Autodesk Inventor part; units mm, degrees
ref_plane "YZ Plane" through (0, 0, 0) normal (1, 0, 0) x (0, 1, 0)
ref_plane "XZ Plane" through (0, 0, 0) normal (0, 1, 0) x (-1, 0, 0)
ref_plane "XY Plane" through (0, 0, 0) normal (0, 0, 1) x (1, 0, 0)
sketch "Sketch1" plane through (0, 0, 0) normal (0, 1, 0) x (-1, 0, 0)
  line L0 (-26, 23.75) -> (26, 23.75)
  line L1 (26, 23.75) -> (26, -23.75)
  line L2 (26, -23.75) -> (-26, -23.75)
  line L3 (-26, -23.75) -> (-26, 23.75)
  line L4 (-26, 23.75) -> (26, -23.75) construction
  line L5 (26, 23.75) -> (-26, -23.75) construction
  point P0 (0, 0)
  dimension "d0" = 52
  dimension "d1" = 47.5
extrude "Extrusion1" add sketch "Sketch1" along normal blind 3
fillet "Fillet1" radius 5 2 edges at (26, 1.5, 23.75) (-26, 1.5, 23.75)
sketch "Sketch2" plane through (0, 3, 0) normal (0, 1, 0) x (1, 0, 0)
  arc A0 (-26, -18.75) -> (-21, -23.75) centre (-21, -18.75) ccw
  line L0 (-21, -23.75) -> (21, -23.75)
  arc A1 (21, -23.75) -> (26, -18.75) centre (21, -18.75) ccw
  line L1 (26, -18.75) -> (26, 23.75)
  line L2 (26, 23.75) -> (-26, 23.75)
  line L3 (-26, 23.75) -> (-26, -18.75)
  line L4 (29, 26.75) -> (29, -18.75)
  arc A2 (21, -26.75) -> (29, -18.75) centre (21, -18.75) ccw
  line L5 (21, -26.75) -> (-21, -26.75)
  arc A3 (-29, -18.75) -> (-21, -26.75) centre (-21, -18.75) ccw
  line L6 (-29, -18.75) -> (-29, 26.75)
  line L7 (-29, 26.75) -> (29, 26.75)
  point P0 (0, 0)
  dimension "d5" = 3
extrude "Extrusion2" add sketch "Sketch2" against normal blind 5
sketch "Sketch3" plane through (0, 3, 0) normal (0, 1, 0) x (1, 0, 0)
  line L0 (26, -18.75) -> (26, 23.75)
  line L1 (29, 26.75) -> (26, 26.75)
  line L2 (26, 26.75) -> (26, 23.75)
  line L3 (26, 23.75) -> (29, 23.75)
  line L4 (29, 23.75) -> (29, 26.75)
  line L5 (26, 23.75) -> (21, 23.75)
  line L6 (21, 23.75) -> (21, 18.75)
  line L7 (21, 18.75) -> (26, 18.75)
  line L8 (26, 18.75) -> (26, 23.75)
  line L9 (-29, 26.75) -> (-26, 26.75)
  line L10 (-26, 26.75) -> (-26, 23.75)
  line L11 (-26, 23.75) -> (-29, 23.75)
  line L12 (-29, 23.75) -> (-29, 26.75)
  line L13 (-26, 23.75) -> (-21, 23.75)
  line L14 (-21, 23.75) -> (-21, 18.75)
  line L15 (-21, 18.75) -> (-26, 18.75)
  line L16 (-26, 18.75) -> (-26, 23.75)
  arc A0 (-29, -18.75) -> (-21, -26.75) centre (-21, -18.75) ccw
  line L17 (21, 18.75) -> (-21, 18.75)
  line L18 (-21, 18.75) -> (-21, -18.75)
  line L19 (-21, -18.75) -> (21, -18.75)
  line L20 (21, -18.75) -> (21, 18.75)
  line L21 (-21, -18.75) -> (-26, -18.75)
  line L22 (-26, -18.75) -> (-26, -23.75)
  line L23 (-26, -23.75) -> (-21, -23.75)
  line L24 (-21, -23.75) -> (-21, -18.75)
  line L25 (-21, -18.75) -> (-24.5355, -22.2855)
  line L26 (-21, -18.75) -> (-16, -18.75) construction
  line L27 (21, -18.75) -> (24.5355, -22.2855)
  line L28 (24.5355, -22.2855) -> (-24.5355, -22.2855)
  line L29 (26, 18.75) -> (21, 23.75)
  line L30 (-21, 23.75) -> (-26, 18.75)
  line L31 (22.7678, -20.5178) -> (-22.7678, -20.5178)
  line L32 (23.5, 21.25) -> (-23.5, 21.25)
  point P0 (0, 0)
  dimension "d8" = 3
  dimension "d9" = 3
  dimension "d10" = 5
  dimension "d11" = 5
  dimension "d12" = 3
  dimension "d13" = 3
  dimension "d14" = 5
  dimension "d15" = 5
  dimension "d16" = 37.5
  dimension "d17" = 5
  dimension "d18" = 5
  dimension "d19" = 5
  dimension "d20" = 135
  dimension "d21" = 5
hole "Hole1" at (-23.5, 3, -21.25) at (23.5, 3, -21.25) at (22.7678, 3, 20.5178) at (-22.7678, 3, 20.5178) direction (0, -1, 0) diameter 2.2 end through all countersink diameter 4 countersink angle 90
fillet "Fillet2" radius 3 5 edges at (26.6569, 3, 24.4069) (0, 3, 26.75) (-26.6569, 3, 24.4069) (-29, 3, -4) (29, 3, -4)
thicken "Thicken1" operation add thickness 3 both sides no extend neighbours yes toward (0, 0, 1) faces at (8.6667, -0.3333, -26.75)
properties part number "Closing_Stepper_2"
Input: part model. Units: mm. Frame: model coordinates. A direction names the side the tool comes from. Round coordinates to 2 decimals unless told otherwise and drop trailing zeros. Loops run counter-clockwise (first coordinate to the right, second up) from the corner with the lowest first, then second, coordinate; pieces in that order, holes last. Notation, with made-up numbers: M -24,2 L 28,2 A16 cw 28,10 Z; hole C 51.5,66 d2. An arc over 180 degrees is marked long. Answer as CSV lines item,"result". Start each with the question number.
(1) First-contact query: pin 1 (2.5 mm diameter, centred on x = 22.77, z = 20.52, fed in from +Y); pin 2 (0.6 mm diameter, centred on x = 0.5, y = -1.5, fed in from -Z); pin 3 (1 mm diameter, centred on x = -20.5, z = 10.5, fed in from -Y). Flat tips, straight axial feed; report the tip coordinate or a pass-through.
(2) Section C-C, the plane y = 0.9. Output: boundary loops of the cut face in (x, z), plus the area to 3 significant figures.
(3) Section B-B, the plane x = 15. Output: boundary loops of the cut face in (y, z).
(4) Section D-D, the plane z = -14. Output: boundary loops of the cut face in (x, y).
(5) Draft query along X for faces 3 (the cylindrical face through (-28.1, 2.14, -2.2)), 4 (the flat face through (0, -1, 23.75)), 5 (the flat face through (29, -1, -3)). Return one class per face: released by +X, released by -X, zero draft, split by the parting line, or undercut.
(6) Section A-A, the plane z = -21.25. Output: boundary loops of the cut face in (x, y), plus the area to 3 significant figures.
(7) Line query: line 1 (X direction, y = 0.45, z = -21.25); line 2 (X direction, y = -1.55, z = -4); line 3 (Y direction, x = -1, z = -7). Output: solid intervals per line, ascending. Write a range as [from, to].
(8) Reachability of faces 1 (the flat face through (0, 2, -23.75)), 2 (the cylindrical face through (-24.57, -0.99, 22.25)) from +Z, -Z, +X, -X, +Y, -Y: full face, straight path, thin tool, end or side. Return the list, or none.
Values found:
1,pin 1,"stops at y = 2.25"
1,pin 2,"stops at z = 23.75"
1,pin 3,"stops at y = 0"
2,outline,"M -28.86,-23.75 L 28.86,-23.75 L 28.86,18.75 A7.86 ccw 21,26.61 L -21,26.61 A7.86 ccw -28.86,18.75 Z; hole C -23.5,-21.25 d2.2; hole C -22.77,20.52 d2.2; hole C 22.77,20.52 d2.2; hole C 23.5,-21.25 d2.2"
2,area,"2,870 mm²"
3,outline,"M -2,23.75 L 0,23.75 L 0,-23.75 L 3,-23.75 L 3,23.75 A3 ccw 0,26.75 L -2,26.75 Z"
4,outline,"M -29,-2 L -26,-2 L -26,0 L 26,0 L 26,-2 L 29,-2 L 29,0 A3 ccw 26,3 L -26,3 A3 ccw -29,0 Z"
5,face 3,"released by -X"
5,face 4,"undercut"
5,face 5,"released by +X"
6,outline,"M -29,-2 L -26,-2 L -26,0 L -24.6,0 L -24.6,2.1 L -25.5,3 L -26,3 A3 ccw -29,0 Z; M -22.4,0 L 22.4,0 L 22.4,2.1 L 21.5,3 L -21.5,3 L -22.4,2.1 Z; M 24.6,0 L 26,0 L 26,-2 L 29,-2 L 29,0 A3 ccw 26,3 L 25.5,3 L 24.6,2.1 Z"
6,area,"167 mm²"
7,line 1,"x = [-28.97, -24.6], [-22.4, 22.4], [24.6, 28.97]"
7,line 2,"x = [-29, -26], [26, 29]"
7,line 3,"y = [0, 3]"
8,face 1,"-Z, +X, -X, +Y, -Y"
8,face 2,"-Z, -Y"
